Autodesk Fusion 360 part; units mm, degrees
sketch "スケッチ1" plane through (0, 0, 0) normal (0, 0, 1) x (1, 0, 0)
  line L0 (0, 101) -> (0, -101)
  line L1 (208, -101) -> (208, 101)
  line L2 (29, -5) -> (179, -5)
  line L3 (16, -101) -> (16, -18)
  line L4 (0, -101) -> (16, -101)
  arc A0 (29, -5) -> (16, -18) centre (29, -18) ccw
  line L5 (192, -18) -> (192, -101)
  line L6 (192, -101) -> (208, -101)
  arc A1 (192, -18) -> (179, -5) centre (179, -18) ccw
  line L7 (179, 5) -> (29, 5)
  line L8 (16, 18) -> (16, 101)
  arc A2 (16, 18) -> (29, 5) centre (29, 18) ccw
  line L9 (16, 101) -> (0, 101)
  line L10 (192, 101) -> (192, 18)
  arc A3 (179, 5) -> (192, 18) centre (179, 18) ccw
  line L11 (208, 101) -> (192, 101)
extrude "押し出し1" add sketch "スケッチ1" along normal blind 100
The listing builds one solid part. Answer for the finished solid, in the listing's coordinates (mm). A direction names the side the tool comes from. Coordinates: 2 decimals unless noted, no trailing zeros. Write each loop counter-clockwise with the first axis right and the second up, starting at its lowest first coordinate (ties: lowest second). Pieces come first, ordered by that corner, then holes. Notation, with made-up numbers: (-14.75, 43) -> (1.25, 43) arc R27 ccw to (1.25, 73) -> close; hole circle Ø11 at (47, 79). An arc over 180 degrees is marked (long way). One line per question, with ' | ' between items.
1. Straight lines are drawn through the part: line 1 (X direction, y = -52.5, z = 42.5); line 2 (Y direction, x = 154.5, z = 18); line 3 (Y direction, x = 189.5, z = 95). For each, find the intervals that lie inside material, in ascending order.
Verdict:
line 1: x = 0 to 16, 192 to 208 | line 2: y = -5 to 5 | line 3: y = -10.34 to 10.34
2. Which of the six approach directions +Z, -Z, +X, -X, +Y, -Y give full straight-line access (tool end or side, diameter ignored) to faces 1 (the cylindrical face through (19.909, 8.707, 49.3)), 2 (the flat face through (0, 1, 49)), 3 (the cylindrical face through (188.091, -8.707, 49.3))?
Verdict:
face 1: +Z, -Z, +Y | face 2: +Z, -Z, -X, +Y, -Y | face 3: +Z, -Z, -Y
3. Given pin 1 Ø6 at (x, y) = (132.5, -10.5) entering from -Z; pin 2 Ø6 at (x, z) = (50, 30.5) entering from +Y, each flat-ended and moving along its own axis, determine where each tip first touches the part or whether it passes through.
Verdict:
pin 1: passes through | pin 2: stops at y = 5
4. Section C-C (x = 155) is taken. Determine the outline of the cut face in (y, z).
Verdict:
outline: (-5, 0) -> (5, 0) -> (5, 100) -> (-5, 100) -> close
5. Section A-A (y = -83) is taken. Determine the outline of the cut face in (x, z), and give its area (3 significant figures).
Verdict:
outline: (0, 0) -> (16, 0) -> (16, 100) -> (0, 100) -> close; (192, 0) -> (208, 0) -> (208, 100) -> (192, 100) -> close | area: 3,200 mm^2
6. Section B-B (z = 80) is taken. Determine the outline of the cut face in (x, y).
Verdict:
outline: (0, -101) -> (16, -101) -> (16, -18) arc R13 cw to (29, -5) -> (179, -5) arc R13 cw to (192, -18) -> (192, -101) -> (208, -101) -> (208, 101) -> (192, 101) -> (192, 18) arc R13 cw to (179, 5) -> (29, 5) arc R13 cw to (16, 18) -> (16, 101) -> (0, 101) -> close
